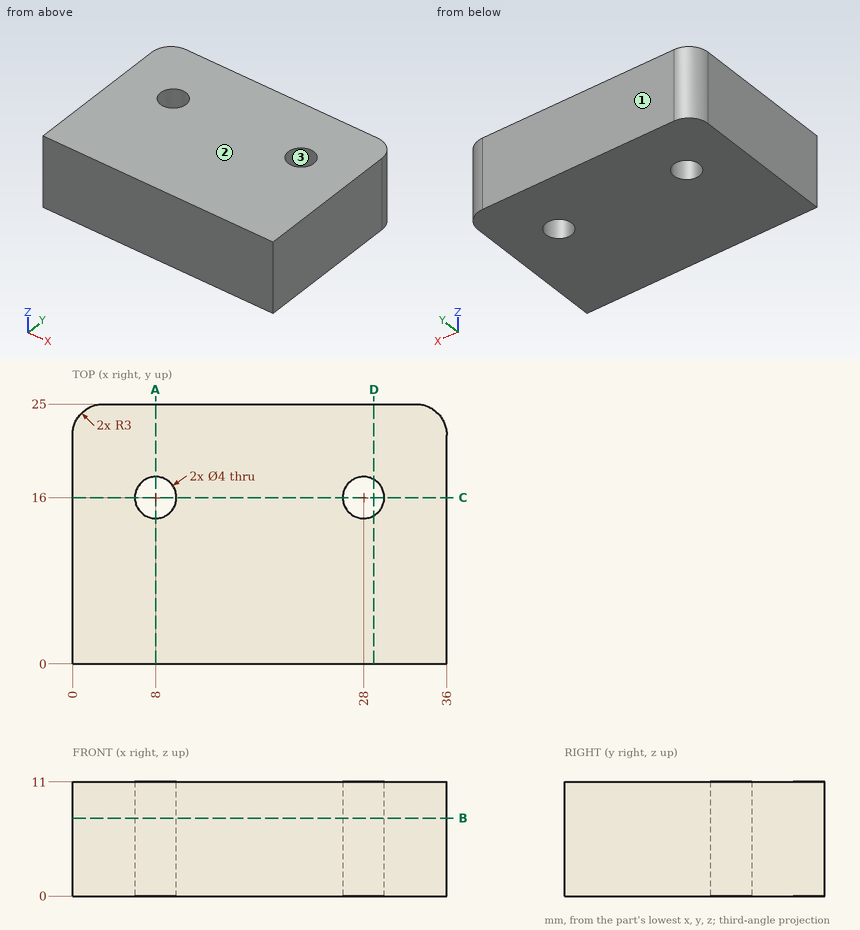
Study the drawing (mm; zero at the part's minimum x, y, z) and answer. Give positions to 0.01 mm unless a question says otherwise; leave off trailing zeros. Write each loop counter-clockwise with the first axis right and the second up, starting at its lowest first coordinate (ties: lowest second). Pieces come first, ordered by that corner, then holes. Notation, with made-up numbers: (62.5, 19) -> (117.5, 19) arc R33 ccw to (117.5, 50) -> close; hole circle Ø10 at (71, 47). An arc over 180 degrees is marked (long way). Answer as a JSON object with one key per item and string values. Group by question number.
1) Find section C-C (y = 16). Write down the section's boundary in (x, z), and give its area (3 significant figures).
2) Find section A-A (x = 8). Write down the section's boundary in (y, z).
3) Consider L1, parallel to Y at x = 28, z = 3; L2, parallel to Y at x = 27, z = 7; L3, parallel to X at y = 22.75, z = 10.25. Determine where each line is inside the solid, lowest interval first. Write a range as from..to.
4) Find section B-B (z = 7.5). Write down the section's boundary in (x, y).
5) Find section D-D (x = 29). Write down the section's boundary in (y, z), and give its area (3 significant figures).
6) The mould has two halves that part along Y. Classify the marked faces 1, 2 and 3: +Y half, -Y half, draft (parallel to the pull), parting line (faces both ways), or undercut.
Values follow:
{
 "1": {"outline": "(0, 0) -> (6, 0) -> (6, 11) -> (0, 11) -> close; (10, 0) -> (26, 0) -> (26, 11) -> (10, 11) -> close; (30, 0) -> (36, 0) -> (36, 11) -> (30, 11) -> close", "area": "308 mm2"},
 "2": {"outline": "(0, 0) -> (14, 0) -> (14, 11) -> (0, 11) -> close; (18, 0) -> (25, 0) -> (25, 11) -> (18, 11) -> close"},
 "3": {"L1": "y = 0..14, 18..25", "L2": "y = 0..14.27, 17.73..25", "L3": "x = 0.1..35.9"},
 "4": {"outline": "(0, 0) -> (36, 0) -> (36, 22) arc R3 ccw to (33, 25) -> (3, 25) arc R3 ccw to (0, 22) -> close; hole circle Ø4 at (8, 16); hole circle Ø4 at (28, 16)"},
 "5": {"outline": "(0, 0) -> (14.27, 0) -> (14.27, 11) -> (0, 11) -> close; (17.73, 0) -> (25, 0) -> (25, 11) -> (17.73, 11) -> close", "area": "237 mm2"},
 "6": {"face 1": "+Y half", "face 2": "draft", "face 3": "undercut"}
}
